from build123d import *

# Parameters (mm, degrees)
SKETCH_1_W               = 50
SKETCH_1_H               = 50
EXTRUDE_1_DEPTH          = 125
CUT_EXTRUDE_1_REACH      = 138.931
CUT_EXTRUDE_1_END_RADIUS = 13.682408883
SKETCH_4_R               = 2.5


with BuildPart() as part:
    # 草图1 → 凸台-拉伸1 (new body)
    with BuildSketch(Plane(origin=(0, 0, 0), x_dir=(1, 0, 0), z_dir=(0, 1, 0))):
        Rectangle(SKETCH_1_W, SKETCH_1_H)
    extrude(amount=EXTRUDE_1_DEPTH)

    # 草图3 → 切除-旋转1 (revolve, cut)
    with BuildSketch(Plane.XY, mode=Mode.PRIVATE) as cut_revolve_1_sk:
        Polygon((0, 125), (0, 25), (5, 25), (13.682408883, 74.240387651), (13.682408883, 125), align=None)
    revolve(cut_revolve_1_sk.sketch.rotate(Axis((0, 125, 0), (0, -1, 0)), 180), axis=Axis((0, 125, 0), (0, -1, 0)), mode=Mode.SUBTRACT)

    # 切除-拉伸1: up to this cylinder (the profile starts outside it)
    cut_extrude_1_end = Plane(origin=(0, 86.74, 0), z_dir=(0, 1, 0)) * Cylinder(CUT_EXTRUDE_1_END_RADIUS, 306.226817767, mode=Mode.PRIVATE)
    # 草图4 → 切除-拉伸1 (cut, up to the surface)
    with BuildSketch(Plane.ZY.offset(25), mode=Mode.PRIVATE) as cut_extrude_1_sk1:
        with Locations((0, 86.74)):
            Circle(SKETCH_4_R)
    cut_extrude_1_tool1 = extrude(cut_extrude_1_sk1.sketch, amount=-CUT_EXTRUDE_1_REACH, mode=Mode.PRIVATE) - cut_extrude_1_end
    add(cut_extrude_1_tool1.solids().sort_by_distance((-25, 86.74, 0))[0], mode=Mode.SUBTRACT)


solid = part.part
For this review, take the finished solid that the model builds, in its own axes (mm). A direction names the side the tool comes from. Give positions to 0.01 mm unless a question says otherwise; leave off trailing zeros. Order: outer loops, then holes, each group sorted by start corner. A loop starts at its lowest first (then second) coordinate and runs counter-clockwise, first axis right, second up. Notation, with made-up numbers: (27, -14) - (81, -14) arc R11 cw to (81, 2) - close; hole circle Ø11 at (-16, 10). An arc over 180 degrees is marked (long way). Answer as a JSON object with one key per item and string values. Group by question number.
Item 1: Take a section at A-A on z = 0. Give the boundary of the cut face in (x, y), and give its area (3 significant figures).
Item 2: Clearance check with flat-ended pins moving along their axes: pin 1 Ø5 at (x, z) = (-8, 17.5) entering from -Y; pin 2 Ø5 at (x, z) = (-1.5, -1) entering from +Y. State where each tip first meets the part, or that it passes through.
Item 3: Take a section at D-D on y = 86.74. Give the boundary of the cut face in (x, z).
Item 4: Draft analysis for pull direction Z (two halves, no side actions). For faces 4 (the conical face through (1.22, 49.96, -9.32)), 5 (the flat face through (0, 0, 0)), 6 (the flat face through (0, 62, -25)), 7 (the flat face through (0, 62, 25)), state which applies: pulls with the +Z half, pulls with the -Z half, needs draft (parallel to the pull), parting line crosses it, or undercut.
Item 5: Take a section at C-C on x = 0. Give the boundary of the cut face in (y, z).
Item 6: Take a section at B-B on y = 103.5. Give the boundary of the cut face in (x, z).
Item 7: Wall thickness on line 1 along Z through (x, y) = (-21, 86.74); line 2 along Z through (x, y) = (0, 101); line 3 along X through (y, z) = (119.5, 8.5): over which ranges is each line inside the solid? List them lowest first.
Item 8: Machinability: for faces 1 (the flat face through (0, 25, 0)), 2 (the cylindrical face through (-19.3, 84.3, -0.54)), 3 (the flat face through (-11, 125, -11)), which of the approach directions +Z, -Z, +X, -X, +Y, -Y give a long, thin tool a straight path to every point of the face, cutting with its end or side? Answer none if there is none.
Reported:
{
 "1": {"outline": "(-25, 0) - (25, 0) - (25, 125) - (13.68, 125) - (13.68, 74.24) - (5, 25) - (-5, 25) - (-13.68, 74.24) - (-13.68, 84.24) - (-25, 84.24) - close; (-25, 89.24) - (-13.68, 89.24) - (-13.68, 125) - (-25, 125) - close", "area": "3,880 mm^2"},
 "2": {"pin 1": "y = 0", "pin 2": "y = 25"},
 "3": {"outline": "(-25, -25) - (25, -25) - (25, 25) - (-25, 25) - (-25, 2.5) - (-13.45, 2.5) arc R13.68 cw (long way) to (-13.45, -2.5) - (-25, -2.5) - close"},
 "4": {"face 4": "undercut", "face 5": "needs draft", "face 6": "pulls with the -Z half", "face 7": "pulls with the +Z half"},
 "5": {"outline": "(0, -25) - (125, -25) - (125, -13.68) - (74.24, -13.68) - (25, -5) - (25, 5) - (74.24, 13.68) - (125, 13.68) - (125, 25) - (0, 25) - close"},
 "6": {"outline": "(-25, -25) - (25, -25) - (25, 25) - (-25, 25) - close; hole circle Ø27.36 at (0, 0)"},
 "7": {"line 1": "-25 to -2.5, 2.5 to 25", "line 2": "-25 to -13.68, 13.68 to 25", "line 3": "-25 to -10.72, 10.72 to 25"},
 "8": {"face 1": "+Y", "face 2": "-X", "face 3": "+Z, -Z, +X, -X, +Y"}
}
